Geometry: see drawing. Coordinates: mm, zero at the bounding-box minimum. A direction names the side the tool comes from. Give positions to 0.01 mm unless a question says otherwise; leave off trailing zeros. Write each loop counter-clockwise with the first axis right and the second up, starting at its lowest first coordinate (ties: lowest second). Pieces come first, ordered by that corner, then holes. Notation, with made-up numbers: (76.25, 39) -> (92.25, 39) arc R14 ccw to (92.25, 59) -> close; hole circle Ø9 at (63, 81). An arc over 180 degrees is marked (long way). Use CSV: the item, a comma, the result in double quotes. Start each with the question number.
1) Set-up query: the marked faces 1, 2 and 3. Return all of +Z, -Z, +X, -X, +Y, -Y with unobstructed straight access to the full face (end or side cutting, diameter ignored); none if empty.
2) Draft query along Z for the marked faces 4, 5 and 6. Return one class per face: pulls with the +Z half, pulls with the -Z half, needs draft (parallel to the pull), parting line crosses it, or undercut.
3) Section B-B (x = 69.85). Output: boundary loops of the cut face in (y, z), plus the area to 3 significant figures.
4) Section D-D (x = 10). Output: boundary loops of the cut face in (y, z), plus the area to 3 significant figures.
5) Contact query for flat-ended pins moving along their axis: P1, Ø7.5, axis at x = 69.85, z = 12.7, coming from the +Y side; P2, Ø1, axis at y = 30, z = 6, coming from the +X side; P3, Ø6.5, axis at x = 75.5, z = 14.5, coming from the +Y side; P4, Ø4.5, axis at y = 29.5, z = 12.5, coming from the -X side. Output: stop coordinate, or through.
6) Material intervals for line 1 (X direction, y = 6.5, z = 12.7); line 2 (Z direction, x = 12.7, y = 10.5); line 3 (Y direction, x = 21, z = 16.25), sorted ascending. Write a range as [from, to].
7) Section A-A (z = 12.7). Count the separate pieces of the cut face and the enclosed holes in it, plus the area to 3 significant figures.
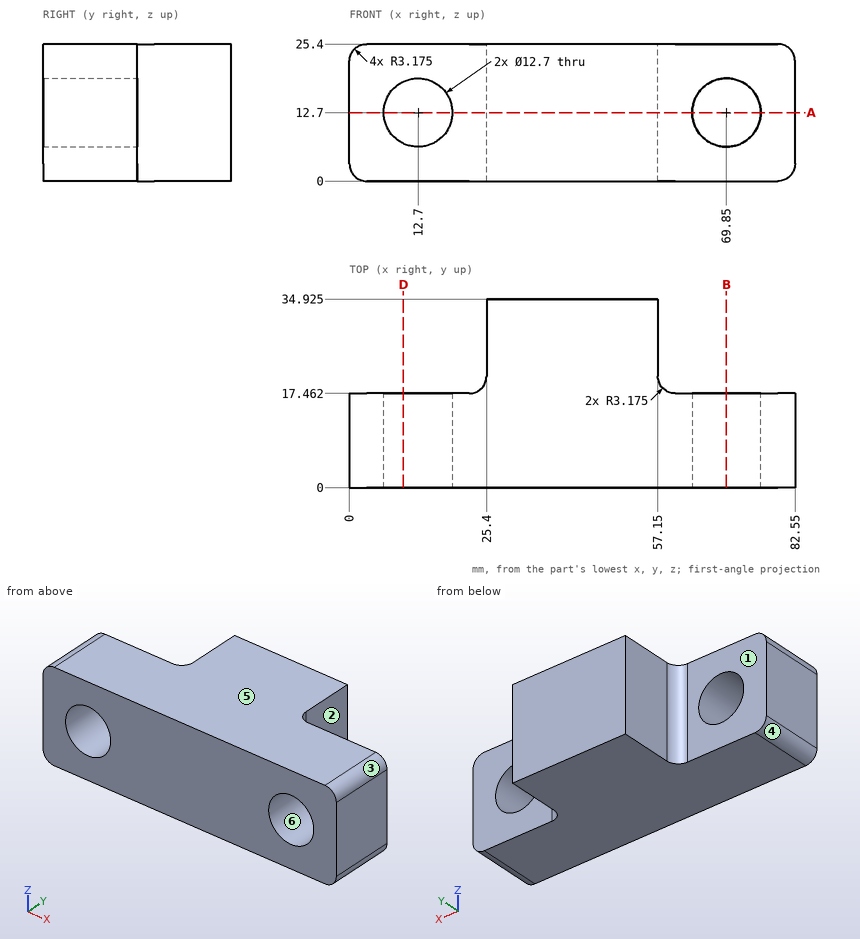
Answers follow:
1,face 1,"+Z, -Z, -X, +Y"
1,face 2,"+Z, -Z, +X, +Y"
1,face 3,"+Z, +X, +Y, -Y"
2,face 4,"pulls with the -Z half"
2,face 5,"pulls with the +Z half"
2,face 6,"undercut"
3,outline,"(0, 0) -> (17.46, 0) -> (17.46, 6.35) -> (0, 6.35) -> close; (0, 19.05) -> (17.46, 19.05) -> (17.46, 25.4) -> (0, 25.4) -> close"
3,area,"222 mm^2"
4,outline,"(0, 0) -> (17.46, 0) -> (17.46, 6.95) -> (0, 6.95) -> close; (0, 18.45) -> (17.46, 18.45) -> (17.46, 25.4) -> (0, 25.4) -> close"
4,area,"243 mm^2"
5,P1,"passes through"
5,P2,"stops at x = 57.15"
5,P3,"stops at y = 17.46"
5,P4,"stops at x = 25.4"
6,line 1,"x = [0, 6.35], [19.05, 63.5], [76.2, 82.55]"
6,line 2,"z = [0, 6.35], [19.05, 25.4]"
6,line 3,"y = [0, 17.46]"
7,separate pieces,"3"
7,enclosed holes,"0"
7,area,"1,560 mm^2"
